```python
from build123d import *

# Parameters (mm, degrees)
CUT_EXTRUDE1_DEPTH = 6.35
CHAMFER1_SIZE      = 0.9652
CHAMFER2_SIZE      = 0.9652


with BuildPart() as part:
    # Sketch2 → Revolve1 (revolve)
    with BuildSketch(Plane.XY):
        Polygon((0, 41.275), (7.14375, 41.275), (7.14375, 31.75), (8.6741, 31.75), (8.6741, 29.3624), (4.7625, 29.3624), (4.7625, 0), (0, 0), align=None)
    revolve(axis=Axis((0, 0, 0), (0, 1, 0)))

    # Sketch3 → Cut-Extrude1 (cut)
    with BuildSketch(Plane(origin=(0, 41.275, 0), x_dir=(1, 0, 0), z_dir=(0, 1, 0))):
        Polygon((4.59005011, 0), (2.295025055, 3.9751), (-2.295025055, 3.9751), (-4.59005011, 0), (-2.295025055, -3.9751), (2.295025055, -3.9751), align=None)
    extrude(amount=-CUT_EXTRUDE1_DEPTH, mode=Mode.SUBTRACT)

    # Chamfer1
    chamfer1_edges = [part.edges().sort_by_distance(p)[0] for p in [
        (-7.14375, 41.275, 0),
    ]]
    chamfer(chamfer1_edges, length=CHAMFER1_SIZE)

    # Chamfer2
    chamfer2_edges = [part.edges().sort_by_distance(p)[0] for p in [
        (-4.7625, 0, 0),
    ]]
    chamfer(chamfer2_edges, length=CHAMFER2_SIZE)


solid = part.part
```
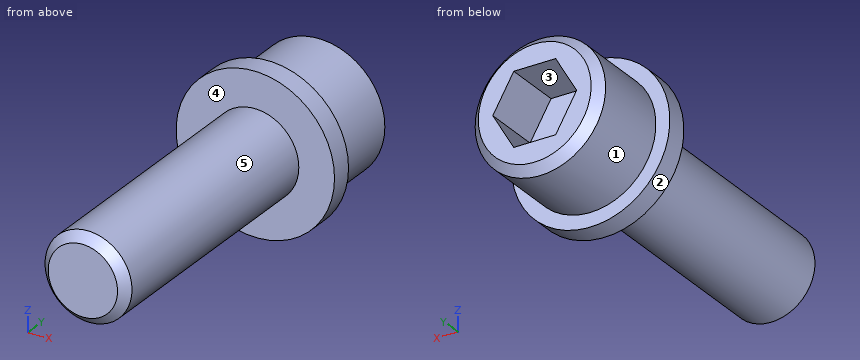
Here's how the part is built. I have some questions about the finished solid (model axes, mm). Face numbers are marked on the shaded views. A direction names the side the tool comes from. Coordinates: 2 decimals unless noted, no trailing zeros. Loops run counter-clockwise (first coordinate to the right, second up) from the corner with the lowest first, then second, coordinate; pieces in that order, holes last. Notation, with made-up numbers: (-21.75, 60) - (7.25, 60) arc R25 cw to (7.25, 96) - close; hole circle Ø7 at (-8.75, 89.5). An arc over 180 degrees is marked (long way). Return JSON: item names as keys, results as strings. Group by question number.
Item 1: Will these pins go through, and if not, where does the flat tip stop? P1, Ø1.4, axis at x = 0.5, y = 37.5, coming from the +Z side; P2, Ø5, axis at y = 35.5, z = 4.5, coming from the -X side; P3, Ø8, axis at y = 12, z = 3, coming from the +X side.
Item 2: If we section it at C-C on y = 34.5: Write out the boundary of the cut face in (x, z).
Item 3: On a 3-axis mill with a long thin cutter (end or side, diameter ignored), from which of +Z, -Z, +X, -X, +Y, -Y can I reach the whole of each face in a straight line? I mean the marked faces 1 and 2. Say none if no direction works.
Item 4: I need wall thicknesses on line 1 (Y direction, x = -3, z = -1.5) (3 decimals); line 2 (Y direction, x = 5.5, z = -1.75) (3 decimals); line 3 (Z direction, x = 0, y = 15). Which ranges of each line are inside material? Lowest first, please. Write a range as from..to.
Item 5: We'd pull the mould along Z, two halves only. Please class the marked faces 3, 4 and 5: +Z half, -Z half, draft (parallel to the pull), parting line (faces both ways), or undercut.
Item 6: If we section it at B-B on y = 9: Write out the boundary of the cut face in (x, z) (1 decimal).
Calculated:
{
 "1": {"P1": "stops at z = 7.14", "P2": "stops at x = -6.86", "P3": "stops at x = 4.76"},
 "2": {"outline": "circle Ø14.29 at (0, 0)"},
 "3": {"face 1": "+Y", "face 2": "+Y, -Y"},
 "4": {"line 1": "y = 0..34.925", "line 2": "y = 29.362..41.275", "line 3": "z = -4.76..4.76"},
 "5": {"face 3": "undercut", "face 4": "draft", "face 5": "parting line"},
 "6": {"outline": "circle Ø9.5 at (0, 0)"}
}
